Source: CAD feature listing. Evaluate the final solid. Frame: model axes, mm. A direction names the side the tool comes from. Coordinates: 2 decimals unless noted, no trailing zeros. Loops run counter-clockwise (first coordinate to the right, second up) from the corner with the lowest first, then second, coordinate; pieces in that order, holes last.
from build123d import *
from build123d.topology import SkipClean

# Parameters (mm, degrees)
SKETCH_1_R          = 4
SKETCH_1_R_2        = 3
EXTRUDE_1_DEPTH     = 25
SKETCH_3_R          = 7.5
EXTRUDE_2_DEPTH     = 10
SKETCH_4_R          = 10
EXTRUDE_3_DEPTH     = 13
SKETCH_6_R          = 4
CUT_EXTRUDE_1_DEPTH = 28


with BuildPart() as part:
    # Эскиз1 → Бобышка-Вытянуть1 (new body)
    with BuildSketch(Plane(origin=(0, 0, 0), x_dir=(1, 0, 0), z_dir=(0, 1, 0))):
        with Locations(Location((0, 0, 0), (0, 0, 270))):
            Circle(SKETCH_1_R)
        with Locations(Location((0, 0, 0), (0, 0, 270))):
            Circle(SKETCH_1_R_2, mode=Mode.SUBTRACT)
    extrude(amount=EXTRUDE_1_DEPTH)

    # Эскиз2 → Повернуть1 (revolve)
    with BuildSketch(Plane.XY, mode=Mode.PRIVATE) as revolve_1_sk:
        with BuildLine():
            Line((0, 25), (0, 40))
            ThreePointArc((0, 40), (5.303300859, 37.803300859), (7.5, 32.5))
            Line((7.5, 32.5), (7.5, 25))
            Line((7.5, 25), (0, 25))
        make_face()
    revolve(revolve_1_sk.sketch.rotate(Axis((0, 25, 0), (0, 1, 0)), 90), axis=Axis((0, 25, 0), (0, 1, 0)))

    # Эскиз3 → Бобышка-Вытянуть2 (add)
    with SkipClean():  # the faces are left unmerged after this step: merging them gives an invalid solid
        with BuildSketch(Plane.XY):
            with Locations((0, 32.5)):
                Circle(SKETCH_3_R)
        extrude(amount=EXTRUDE_2_DEPTH)

    # Эскиз4 → Бобышка-Вытянуть3 (add)
    with SkipClean():  # the faces are left unmerged after this step: merging them gives an invalid solid
        with BuildSketch(Plane.XY.offset(10)):
            with Locations(Location((0, 32.5, 0), (0, 0, 180))):
                Circle(SKETCH_4_R)
        extrude(amount=EXTRUDE_3_DEPTH)

    # Эскиз5 → Повернуть3 (revolve)
    with SkipClean():  # the faces are left unmerged after this step: merging them gives an invalid solid
        with BuildSketch(Plane(origin=(0, 0, 0), x_dir=(0, 0, -1), z_dir=(1, 0, 0)), mode=Mode.PRIVATE) as revolve_3_sk:
            Polygon((-26.75, 24.5), (-26.75, 26.5), (-25.75, 26.5), (-25.75, 23.75), (-25, 23), (-23.75, 23), (-23.75, 23.5), (-23, 23.5), (-23, 28.5), (-27.75, 28.5), (-27.75, 24.5), align=None)
        revolve(revolve_3_sk.sketch.rotate(Axis((0, 32.5, 23), (0, 0, 1)), 270), axis=Axis((0, 32.5, 23), (0, 0, 1)))

    # Эскиз6 → Вырез-Вытянуть1 (cut)
    with SkipClean():  # the faces are left unmerged after this step: merging them gives an invalid solid
        with BuildSketch(Plane.XY.offset(27.75)):
            with Locations(Location((0, 32.5, 0), (0, 0, 180))):
                Circle(SKETCH_6_R)
        extrude(amount=-CUT_EXTRUDE_1_DEPTH, mode=Mode.SUBTRACT)


solid = part.part
Q1. Draft query along Z for faces 5 (the cylindrical face through (0.9, 12.32, 2.86)), 6 (the flat face through (-4, 34, 27.75)), 7 (the cylindrical face through (2.17, 42.26, 16.41)). Return one class per face: +Z half, -Z half, draft (parallel to the pull), parting line (faces both ways), or undercut.
Q2. Section A-A, the plane z = 17. Return the cut outline in (x, y).
Q3. Section B-B, the plane y = 16. Return the cut outline in (x, z).
Q4. Contact query for flat-ended pins moving along their axis: pin 1 Ø5 at (x, z) = (-4.5, 0.5) entering from -Y; pin 2 Ø4 at (x, z) = (5.5, 20.5) entering from +Y; pin 3 Ø3 at (x, z) = (6.5, 16.5) entering from -Y; pin 4 Ø1.5 at (x, y) = (-2, 21.5) entering from -Z. Output: stop coordinate, or through.
Q5. Access query for faces 1 (the flat face through (0, 25, 0)), 2 (the flat face through (3, 0, 1)), 3 (the flat face through (0, 32, -0.25)), 4 (the flat face through (4, 24, 23)). Directions: +Z, -Z, +X, -X, +Y, -Y. A direction counts if a zero-diameter tool reaches every point of the face in a straight line with its end or side. Return the directions, or none.
Q6. Section C-C, the plane z = -1.5. Return the cut outline in (x, y).
Q7. Line query: line 1 along X through (y, z) = (32.5, 13.75); line 2 along Y through (x, z) = (0, 26.05); line 3 along X through (y, z) = (10, 0). Output: solid intervals per line, ascending.
Derived:
1. face 5: undercut
1. face 6: +Z half
1. face 7: draft
2. outline: circle Ø20 at (0, 32.5); hole circle Ø8 at (0, 32.5)
3. outline: circle Ø8 at (0, 0); hole circle Ø6 at (0, 0)
4. pin 1: stops at y = 0
4. pin 2: stops at y = 41.87
4. pin 3: stops at y = 23.84
4. pin 4: stops at z = -3.8
5. face 1: -Y
5. face 2: +Z, -Z, +X, -X, -Y
5. face 3: +Z
5. face 4: none
6. outline: (-7.35, 25) - (-3.71, 25) - (-3.71, 0) - (-2.6, 0) - (-2.6, 25) - (2.6, 25) - (2.6, 0) - (3.71, 0) - (3.71, 25) - (7.35, 25) - (7.35, 32.5) arc R7.35 ccw to (-7.35, 32.5) - close
7. line 1: x = -10 to -4, 4 to 10
7. line 2: y = 26.5 to 28.5, 36.5 to 38.5
7. line 3: x = -4 to -3, 3 to 4
